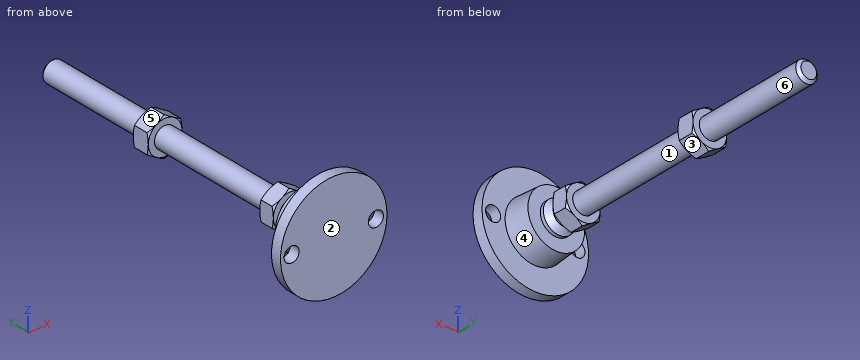
from build123d import *

# Parameters (mm, degrees)
EXTRUDE_1_DEPTH     = 9
EXTRUDE_2_DEPTH     = 10
SKETCH_5_R          = 4.25
CUT_EXTRUDE_1_DEPTH = 7


with BuildPart() as part:
    # Эскиз1 → Повернуть1 (revolve)
    with BuildSketch(Plane.XY, mode=Mode.PRIVATE) as revolve_1_sk:
        Polygon((0, 0), (-30, 0), (-30, 6), (-17, 6), (-16, 20), (-9, 20), (-9, 22), (-6, 25), (-6, 29), (-6, 38), (-6, 186.4), (-4.4, 188), (0, 188), align=None)
    revolve(revolve_1_sk.sketch.rotate(Axis((0, 0, 0), (0, 1, 0)), 180), axis=Axis((0, 0, 0), (0, 1, 0)))  # turned: the seam where the file's is

    # Эскиз2 → Бобышка-Вытянуть1 (add)
    with BuildSketch(Plane(origin=(0, 29, 0), x_dir=(1, 0, 0), z_dir=(0, 1, 0))):
        Polygon((0, 10.969655115), (-9.5, 5.484827557), (-9.5, -5.484827557), (0, -10.969655115), (9.5, -5.484827557), (9.5, 5.484827557), align=None)
    extrude(amount=EXTRUDE_1_DEPTH)

    # Эскиз3 → Бобышка-Вытянуть2 (add)
    with BuildSketch(Plane(origin=(0, 112.2, 0), x_dir=(1, 0, 0), z_dir=(0, 1, 0))):
        Polygon((9.5, 5.484827557), (0, 10.969655115), (-9.5, 5.484827557), (-9.5, -5.484827557), (0, -10.969655115), (9.5, -5.484827557), align=None)
    extrude(amount=EXTRUDE_2_DEPTH)

    # Эскиз4 → Вырез-Повернуть2 (revolve, cut)
    with BuildSketch(Plane.XY, mode=Mode.PRIVATE) as cut_revolve_2_sk:
        Polygon((-18.160254038, 122.2), (-9.5, 122.2), (-18.160254038, 117.2), align=None)
        Polygon((-18.160254038, 112.2), (-18.160254038, 117.2), (-9.5, 112.2), align=None)
        Polygon((-17.294228634, 38), (-17.294228634, 33.5), (-9.5, 38), align=None)
        Polygon((-17.294228634, 33.5), (-17.294228634, 29), (-9.5, 29), align=None)
    revolve(cut_revolve_2_sk.sketch.rotate(Axis((0, 188, 0), (0, -1, 0)), 180), axis=Axis((0, 188, 0), (0, -1, 0)), mode=Mode.SUBTRACT)  # turned: the seam where the file's is

    # Эскиз5 → Вырез-Вытянуть1 (cut, through all)
    with BuildSketch(Plane(origin=(0, 6, 0), x_dir=(1, 0, 0), z_dir=(0, 1, 0))):
        with Locations(Location((-23.75, 0, 0), (0, 0, 180))):  # turned: the seam where the file's is
            Circle(SKETCH_5_R)
        with Locations(Location((23.75, 0, 0), (0, 0, 180))):  # turned: the seam where the file's is
            Circle(SKETCH_5_R)
    extrude(amount=-CUT_EXTRUDE_1_DEPTH, mode=Mode.SUBTRACT)


solid = part.part
For this review, take the finished solid that the model builds, in its own axes (mm). Face numbers are marked on the shaded views. A direction names the side the tool comes from. Give positions to 0.01 mm unless a question says otherwise; leave off trailing zeros. Write each loop counter-clockwise with the first axis right and the second up, starting at its lowest first coordinate (ties: lowest second). Pieces come first, ordered by that corner, then holes. Notation, with made-up numbers: (-1, -18) -> (26, -18) arc R21 ccw to (26, -7) -> close; hole circle Ø1 at (18, 31.25). An arc over 180 degrees is marked (long way). Use CSV: the item, a comma, the result in double quotes.
Q1. To check wall thickness, follow probe 1 along Y at (x, z) = (-7, 7); probe 2 along Z at (x, y) = (23, 3); probe 3 along Z at (x, y) = (23.75, 4). State the ranges of each line that lie inside material, in increasing order. Write a range as [from, to].
Conclusion:
probe 1,"[0, 20]"
probe 2,"[-19.26, -4.18], [4.18, 19.26]"
probe 3,"[-18.33, -4.25], [4.25, 18.33]"
Q2. Tool access review of the marked faces 5 and 6: name each direction out of +Z, -Z, +X, -X, +Y, -Y from which nothing blocks a thin tool from reaching the whole face with its end or side.
Conclusion:
face 5,"+Z, -X, +Y"
face 6,"+Y"
Q3. Take a section at D-D, the plane z = 25.5. Write out the cut boundary in (x, y).
Conclusion:
outline,"(-15.8, 0) -> (15.8, 0) -> (15.8, 6) -> (-15.8, 6) -> close"
Q4. Take a section at A-A, the plane x = 22.5. Write out the cut boundary in (y, z), then the cut area to 3 significant figures.
Conclusion:
outline,"(0, -19.84) -> (6, -19.84) -> (6, -4.06) -> (0, -4.06) -> close; (0, 4.06) -> (6, 4.06) -> (6, 19.84) -> (0, 19.84) -> close"
area,"189 mm2"
Q5. Take a section at C-C, the plane x = -23.75. Write out the cut boundary in (y, z).
Conclusion:
outline,"(0, -18.33) -> (6, -18.33) -> (6, -4.25) -> (0, -4.25) -> close; (0, 4.25) -> (6, 4.25) -> (6, 18.33) -> (0, 18.33) -> close"
Q6. Mouldability with a two-part tool opening along Y and no side actions: class the marked faces 1, 2, 3 and 4 as pulls with the +Y half, pulls with the -Y half, needs draft (parallel to the pull), parting line crosses it, or undercut.
Conclusion:
face 1,"undercut"
face 2,"pulls with the -Y half"
face 3,"needs draft"
face 4,"pulls with the +Y half"
Q7. For P1, Ø3, axis at x = 13, z = -1, coming from the +Y side; P2, Ø7.5, axis at x = -23.75, z = 0, coming from the +Y side; P3, Ø4, axis at y = 24.5, z = -1.5, coming from the +X side; P4, Ø12, axis at y = 43, z = -4.5, coming from the +X side, all flat-tipped, find the tip position at first contact; note any pin that passes through.
Conclusion:
P1,"y = 20"
P2,"through"
P3,"x = 8.39"
P4,"x = 9.5"
Q8. Take a section at B-B, the plane y = 118.5. Write out the cut boundary in (x, z).
Conclusion:
outline,"(-9.5, -5.48) -> (0, -10.97) -> (9.5, -5.48) -> (9.5, 5.48) -> (0, 10.97) -> (-9.5, 5.48) -> close"
